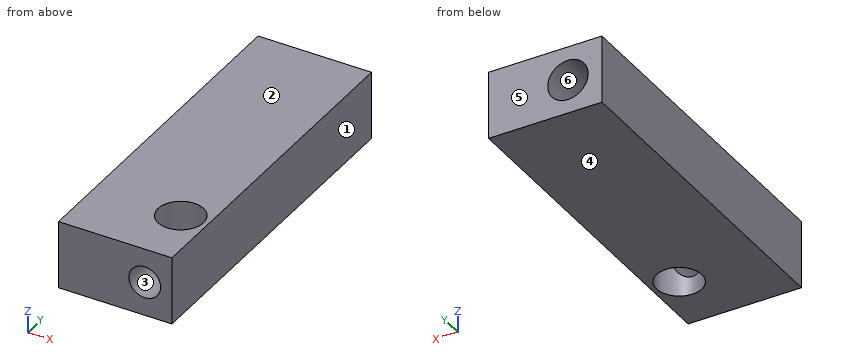
from build123d import *

# Parameters (mm, degrees)
SKETCH1_W                  = 6.35
SKETCH1_H                  = 3.81
BOSS_EXTRUDE1_DEPTH        = 19.05
F_4_40_TAPPED_HOLE1_D      = 2.2606
F_4_40_TAPPED_HOLE1_DEPTH  = 7.62
F_4_40_TAPPED_HOLE1_TIP    = 0.679152758
SKETCH8_R                  = 1.27
CUT_EXTRUDE3_DEPTH         = 20.685
F_2_56_TAPPED_HOLE2_REACH  = 21.406
F_2_56_TAPPED_HOLE2_BORE_R = 0.889


with BuildPart() as part:
    # Sketch1 → Boss-Extrude1 (new body)
    with BuildSketch(Plane(origin=(0, 0, 0), x_dir=(1, 0, 0), z_dir=(0, 1, 0))):
        Rectangle(SKETCH1_W, SKETCH1_H)
    extrude(amount=-BOSS_EXTRUDE1_DEPTH)

    # #4-40 Tapped Hole1
    with Locations(Plane(origin=(0, 0, 0), x_dir=(1, 0, 0), z_dir=(0, 1, 0))):
        with Locations((-1.27, 0)):
            Hole(F_4_40_TAPPED_HOLE1_D / 2, depth=F_4_40_TAPPED_HOLE1_DEPTH)
            with Locations((0, 0, -(F_4_40_TAPPED_HOLE1_DEPTH + F_4_40_TAPPED_HOLE1_TIP / 2))):  # 118° drill point
                Cone(0, F_4_40_TAPPED_HOLE1_D / 2, F_4_40_TAPPED_HOLE1_TIP, mode=Mode.SUBTRACT)

    # Sketch8 → Cut-Extrude3 (cut, through all)
    with BuildSketch(Plane.XY.offset(1.905)):
        with Locations((1.651, -15.60576)):
            Circle(SKETCH8_R)
    extrude(amount=-CUT_EXTRUDE3_DEPTH, mode=Mode.SUBTRACT)

    # #2-56 Tapped Hole2 bore → #2-56 Tapped Hole2 (cut, up to next)
    with BuildSketch(Plane(origin=(0, -19.05, 0), x_dir=(-1, 0, 0), z_dir=(0, -1, 0)), mode=Mode.PRIVATE) as f_2_56_tapped_hole2_sk1:
        with Locations((-1.651, 0)):
            Circle(F_2_56_TAPPED_HOLE2_BORE_R)
    f_2_56_tapped_hole2_tool1 = extrude(f_2_56_tapped_hole2_sk1.sketch, amount=-F_2_56_TAPPED_HOLE2_REACH, mode=Mode.PRIVATE) & part.part
    add(f_2_56_tapped_hole2_tool1.solids().sort_by_distance((1.651, -19.05, 0))[0], mode=Mode.SUBTRACT)


solid = part.part
Input: part model. Units: mm. Frame: model coordinates. Face numbers are marked on the shaded views. A direction names the side the tool comes from. Coordinates: 2 decimals unless noted, no trailing zeros. Loops run counter-clockwise (first coordinate to the right, second up) from the corner with the lowest first, then second, coordinate; pieces in that order, holes last.
Q1. Draft query along Z for the marked faces 1, 2, 3 and 4. Return one class per face: +Z half, -Z half, draft (parallel to the pull), parting line (faces both ways), or undercut.
Q2. Cut plane D-D (x = 2.75). Output: boundary loops of the cut face in (y, z) (3 decimals), then the cut area to 3 significant figures.
Q3. Set-up query: the marked faces 5 and 6. Return all of +Z, -Z, +X, -X, +Y, -Y with unobstructed straight access to the full face (end or side cutting, diameter ignored); none if empty.
Q4. Material intervals for line 1 (X direction, y = -17.6, z = 0) (3 decimals); line 2 (X direction, y = -15.5, z = -0.75) (3 decimals); line 3 (Z direction, x = -1.5, y = -8) (3 decimals), sorted ascending.
Q5. Cut plane C-C (z = 1.4). Output: boundary loops of the cut face in (x, y) (3 decimals).
Q6. Cut plane A-A (y = -5.75). Output: boundary loops of the cut face in (x, z) (3 decimals), then the cut area to 3 significant figures.
Q7. Cut plane B-B (x = 1.25). Output: boundary loops of the cut face in (y, z) (3 decimals), then the cut area to 3 significant figures.
Q8. Contact query for a flat-ended pin moving along its axis: pin 1 (1 mm diameter, centred on x = 2, z = -0.5, fed in from +Y). Output: stop coordinate, or through.
Working result:
1. face 1: draft
1. face 2: +Z half
1. face 3: undercut
1. face 4: -Z half
2. outline: (-19.05, -1.905) - (-16.242, -1.905) - (-16.242, 1.905) - (-19.05, 1.905) - close; (-14.969, -1.905) - (0, -1.905) - (0, 1.905) - (-14.969, 1.905) - close
2. area: 67.7 mm2
3. face 5: +Z, -Z, +X, -X, +Y
3. face 6: +Y
4. line 1: x = -3.175 to 0.762, 2.54 to 3.175
4. line 2: x = -3.175 to 0.385, 2.917 to 3.175
4. line 3: z = -1.905 to -0.442, 0.442 to 1.905
5. outline: (-3.175, -19.05) - (3.175, -19.05) - (3.175, 0) - (-3.175, 0) - close; hole circle Ø2.54 at (1.651, -15.606)
6. outline: (-3.175, -1.905) - (3.175, -1.905) - (3.175, 1.905) - (-3.175, 1.905) - close; hole circle Ø2.261 at (-1.27, 0)
6. area: 20.2 mm2
7. outline: (-19.05, -1.905) - (-16.811, -1.905) - (-16.811, -0.793) - (-19.05, -0.793) - close; (-19.05, 0.793) - (-16.811, 0.793) - (-16.811, 1.905) - (-19.05, 1.905) - close; (-14.401, -1.905) - (0, -1.905) - (0, 1.905) - (-14.401, 1.905) - close
7. area: 59.8 mm2
8. pin 1: stops at y = 0
